from build123d import *

# Parameters (mm, degrees)
F0_W     = 51
F0_H     = 43
F1_DEPTH = 1
F2_W     = 31
F2_H     = 10
F2_W_2   = 29
F2_H_2   = 8
F3_DEPTH = 7
F4_DEPTH = 25
F2_W_3   = 23
F2_H_3   = 1
F2_H_4   = 9.8
F5_DEPTH = 25


with BuildPart() as f1:
    # F0 (on Top) → F1 (new body)
    with BuildSketch(Plane.XY):
        Rectangle(F0_W, F0_H)
    extrude(amount=F1_DEPTH)

    # F2 (on face) → F3 (join)
    with BuildSketch(Plane(origin=(0, 0, 0), x_dir=(1, 0, 0), z_dir=(0, 0, -1))):
        Polygon((-11.5, 19.3), (-11.5, 20.3), (-24.3, 20.3), (-24.3, 14.5), (-23.3, 14.5), (-23.3, 19.3), (-12.5, 19.3), align=None)
        Polygon((19.5, -20.3), (24.3, -20.3), (24.3, 20.3), (11.5, 20.3), (11.5, 19.3), (12.5, 19.3), (23.3, 19.3), (23.3, -19.3), (19.5, -19.3), align=None)
        Polygon((-24.3, -20.3), (-19.5, -20.3), (-19.5, -19.3), (-23.3, -19.3), (-23.3, 1.5), (-24.3, 1.5), align=None)
        with Locations((-1, 1.5)):
            Rectangle(F2_W, F2_H)
        with Locations((-1, 1.5)):
            Rectangle(F2_W_2, F2_H_2, mode=Mode.SUBTRACT)
        Polygon((12.5, 19.3), (11.5, 19.3), (11.5, 9.5), (-11.5, 9.5), (-11.5, 19.3), (-12.5, 19.3), (-12.5, 8.5), (12.5, 8.5), align=None)
    extrude(amount=F3_DEPTH)

    # F4 (cut): a face of the model
    f4_faces = [f1.faces().sort_by_distance(p)[0] for p in [
        (-1, -1.5, 0),
    ]]
    extrude(f4_faces, amount=-F4_DEPTH, mode=Mode.SUBTRACT)

    # F2 (on face) → F5 (cut)
    with BuildSketch(Plane(origin=(0, 0, 0), x_dir=(1, 0, 0), z_dir=(0, 0, -1))):
        with Locations((0, 19.8)):
            Rectangle(F2_W_3, F2_H_3)
        with Locations((0, 14.4)):
            Rectangle(F2_W_3, F2_H_4)
    extrude(amount=-F5_DEPTH, mode=Mode.SUBTRACT)


solid = f1.part
The model under review builds one solid part; all positions refer to its coordinate system, in mm. A direction names the side the tool comes from. Coordinates: 2 decimals unless noted, no trailing zeros. Write each loop counter-clockwise with the first axis right and the second up, starting at its lowest first coordinate (ties: lowest second). Pieces come first, ordered by that corner, then holes. Notation, with made-up numbers: M -40,-22.5 L -12,-22.5 A27 cw -12,11.5 Z; hole C 10.5,57 d2. An arc over 180 degrees is marked long. Put each result on its own line as item: value.
1) Clearance check with flat-ended pins moving along their axes: pin 1 Ø3.5 at (x, z) = (-1.5, -2) entering from +Y; pin 2 Ø2.5 at (x, z) = (4, -2) entering from -Y; pin 3 Ø1.1 at (x, z) = (-23.5, -3) entering from -Y; pin 4 Ø10 at (x, y) = (-8.5, 0.5) entering from +Z. State where each tip first meets the part, or that it passes through.
Computed:
pin 1: stops at y = 3.5
pin 2: stops at y = -9.5
pin 3: stops at y = -20.3
pin 4: stops at z = 1
2) For faces 1 (the flat face through (-23.3, -17, -3)), 2 (the flat face through (-24.3, 9, -3)), 3 (the flat face through (-1, -5.5, -3)), list the 3-axis set-ups (+Z, -Z, +X, -X, +Y, -Y) from which the entire face can be reached by the end or side of a thin tool; tool diameter is ignored.
Computed:
face 1: -Z
face 2: -Z, -X, +Y, -Y
face 3: +Z, -Z
3) Add section A-A on z = -1.25. State how many separate pieces and enclosed holes the cut face has, then the cut area to 3 significant figures.
Computed:
separate pieces: 3
enclosed holes: 1
area: 222 mm2
4) Add section C-C on y = -12. Give the boundary of the cut face in (x, z).
Computed:
outline: M -25.5,0 L -12.5,0 L -12.5,-7 L -11.5,-7 L -11.5,1 L -25.5,1 Z; M 11.5,-7 L 12.5,-7 L 12.5,0 L 23.3,0 L 23.3,-7 L 24.3,-7 L 24.3,0 L 25.5,0 L 25.5,1 L 11.5,1 Z
5) Add section B-B on x = -9.5. Give the boundary of the cut face in (y, z).
Computed:
outline: M -21.5,0 L -20.3,0 L -20.3,1 L -21.5,1 Z; M -9.5,-7 L -8.5,-7 L -8.5,0 L -6.5,0 L -6.5,-7 L -5.5,-7 L -5.5,1 L -9.5,1 Z; M 2.5,-7 L 3.5,-7 L 3.5,0 L 21.5,0 L 21.5,1 L 2.5,1 Z
6) Wall thickness on probe 1 along Y at (x, z) = (-15, -4.25); probe 2 along X at (y, z) = (-16, -0.25); probe 3 along Y at (x, z) = (-9, -5.5): over which ranges is each line inside the solid? List them lowest first. Write a range as [from, to].
Computed:
probe 1: y = [-20.3, -19.3], [-6.5, -5.5], [2.5, 3.5]
probe 2: x = [-24.3, -23.3], [-12.5, -11.5], [11.5, 12.5], [23.3, 24.3]
probe 3: y = [-9.5, -8.5], [-6.5, -5.5], [2.5, 3.5]
7) Add section D-D on y = 7.5. Give the boundary of the cut face in (x, z), then the cut area to 3 significant figures.
Computed:
outline: M -25.5,0 L -24.3,0 L -24.3,-7 L -23.3,-7 L -23.3,0 L 23.3,0 L 23.3,-7 L 24.3,-7 L 24.3,0 L 25.5,0 L 25.5,1 L -25.5,1 Z
area: 65.0 mm2
8) Draft analysis for pull direction Y (two halves, no side actions). For faces 4 (the flat face through (-22, 20.3, -3)), 5 (the flat face through (-1, 2.5, -3)), 6 (the flat face through (0, 5, 1)), state which applies: released by +Y, released by -Y, zero draft, split by the parting line, or undercut.
Computed:
face 4: released by +Y
face 5: undercut
face 6: zero draft
